Print and shaded views of the part. All mm, measured from the part's lowest x, y and z. A direction names the side the tool comes from. Give positions to 0.01 mm unless a question says otherwise; leave off trailing zeros. Loops run counter-clockwise (first coordinate to the right, second up) from the corner with the lowest first, then second, coordinate; pieces in that order, holes last. Notation, with made-up numbers: M 7.25,9.5 L 41.25,9.5 A21 cw 41.25,28.5 Z; hole C 80.5,33 d3. An arc over 180 degrees is marked long. Put each result on its own line as item: value. Start each with the question number.
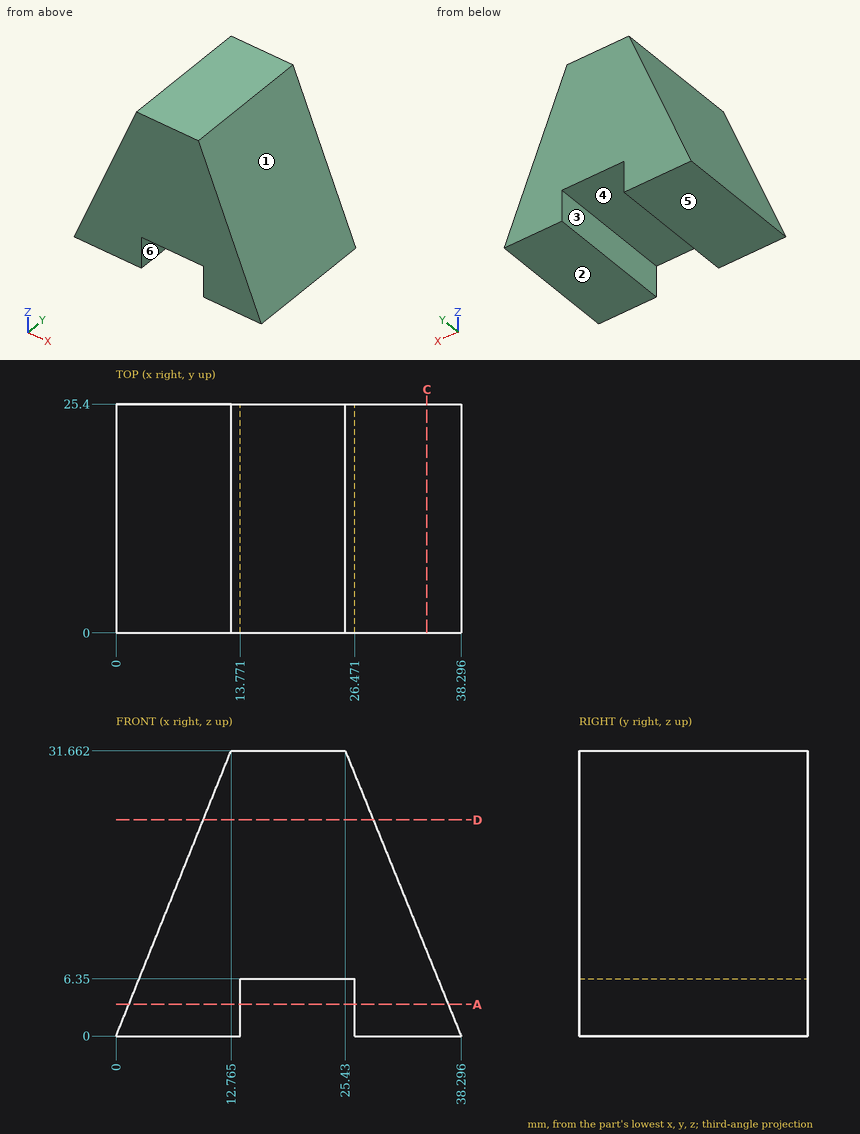
1) Which spindle directions (+Z, -Z, +X, -X, +Y, -Y) get a long thin tool onto all of the face, cutting with end or side? Do the marked faces 5 and 6. Say none if no direction does.
2) Band-saw the part on A-A on z = 3.5. Give the cut face in (x, y).
3) Band-saw the part on C-C on x = 34.5. Give the cut face in (y, z).
4) Band-saw the part on D-D on z = 24. Give the cut face in (x, y).
5) Pin check, flat tips, straight feed: pin 1 Ø5 at (y, z) = (11, 4.5) entering from +X; pin 2 Ø6.5 at (x, y) = (20.5, 10.5) entering from -Z; pin 3 Ø1 at (y, z) = (20.5, 19) entering from -X. Stop position of each tip, or through.
6) Wall check: L1, parallel to Z at x = 18.5, y = 16; L2, parallel to X at y = 22, z = 2 (1 decimal); L3, parallel to X at y = 24.75, z = 3.5 (1 decimal). Give the ranges that are in metal, low to high.
7) Mould opens along X. For the marked faces 1, 2, 3 and 4 say: +X half, -X half, draft (parallel to the pull), parting line (faces both ways), or undercut.
Evaluation:
1. face 5: -Z, +X, -X, +Y, -Y
1. face 6: -Z, +Y, -Y
2. outline: M 1.41,0 L 13.77,0 L 13.77,25.4 L 1.41,25.4 Z; M 26.47,0 L 36.87,0 L 36.87,25.4 L 26.47,25.4 Z
3. outline: M 0,0 L 25.4,0 L 25.4,9.34 L 0,9.34 Z
4. outline: M 9.68,0 L 28.54,0 L 28.54,25.4 L 9.68,25.4 Z
5. pin 1: x = 37.48
5. pin 2: z = 6.35
5. pin 3: x = 7.46
6. L1: 6.35 to 31.66
6. L2: 0.8 to 13.8, 26.5 to 37.5
6. L3: 1.4 to 13.8, 26.5 to 36.9
7. face 1: +X half
7. face 2: draft
7. face 3: undercut
7. face 4: undercut
